```python
from build123d import *

# Parameters (mm, degrees)
CROQUIS1_W              = 30
CROQUIS1_H              = 15
CROQUIS1_W_2            = 12.5
CROQUIS1_H_2            = 12.5
SALIENTE_EXTRUIR1_DEPTH = 10
CHAFL_N1_SIZE           = 10
CHAFL_N1_SIZE2          = 2.679491924
REDONDEO1_R             = 1


with BuildPart() as part:
    # Croquis1 → Saliente-Extruir1 (new body)
    with BuildSketch(Plane(origin=(0, 0, 0), x_dir=(1, 0, 0), z_dir=(0, 1, 0))):
        with Locations((15, 7.5)):
            Rectangle(CROQUIS1_W, CROQUIS1_H)
        with Locations((7.75, 7.5)):
            Rectangle(CROQUIS1_W_2, CROQUIS1_H_2, mode=Mode.SUBTRACT)
    extrude(amount=SALIENTE_EXTRUIR1_DEPTH)

    # Chaflán1
    chafl_n1_edges = [part.edges().sort_by_distance(p)[0] for p in [
        (14, 10, -7.5),
    ]]
    chafl_n1_side = [part.faces().sort_by_distance(p)[0] for p in [
        (18.856382979, 10, -7.5),
    ]]
    chamfer(chafl_n1_edges, length=CHAFL_N1_SIZE, length2=CHAFL_N1_SIZE2, reference=chafl_n1_side[0])

    # Redondeo1
    redondeo1_edges = [part.edges().sort_by_distance(p)[0] for p in [
        (1.5, 5, -13.75),
        (1.5, 5, -1.25),
        (14, 3.660254038, -1.25),
        (14, 3.660254038, -13.75),
        (0, 5, -15),
        (0, 5, 0),
    ]]
    fillet(redondeo1_edges, radius=REDONDEO1_R)


solid = part.part
```
Input: part model. Units: mm. Frame: model coordinates. A direction names the side the tool comes from. Round coordinates to 2 decimals unless told otherwise and drop trailing zeros. Loops run counter-clockwise (first coordinate to the right, second up) from the corner with the lowest first, then second, coordinate; pieces in that order, holes last. Notation, with made-up numbers: (76, 14.5) -> (102, 14.5) arc R12 ccw to (102, 28.5) -> close; hole circle Ø2 at (41.5, -6). An arc over 180 degrees is marked (long way). Use one line per item in the form item = value. Start each with the question number.
Item 1: Section query C-C on y = 0.75. Return the cut outline in (x, z).
Item 2: Mould query, pull axis Z, two halves, no side actions, for faces 1 (the face through (15, 5, -15)), 2 (the face through (30, 5, -7)), 3 (the face through (14, 4, -7)). Classes: pulls with the +Z half, pulls with the -Z half, needs draft (parallel to the pull), parting line crosses it, or undercut.
Item 3: Section query B-B on z = -5.25. Return the cut outline in (x, y).
Item 4: Material intervals for L1, parallel to Z at x = 17, y = 9.25; L2, parallel to X at y = 7, z = -7; L3, parallel to Z at x = 13.5, y = 5, sorted ascending. Write a range as from..to.
Item 5: Section query A-A on x = 5. Return the cut outline in (y, z).
Item 6: Section query D-D on x = 17.75. Return the cut outline in (y, z).
Item 7: Set-up query: faces 4 (the face through (8, 6, -1.25)), 5 (the face through (18, 0, -8)), 6 (the face through (1.801, 5.07, -13.465)). Return all of +Z, -Z, +X, -X, +Y, -Y with unobstructed straight access to the full face (end or side cutting, diameter ignored); none if empty.
Ans:
q1.outline = (0, -14) arc R1 ccw to (1, -15) -> (30, -15) -> (30, 0) -> (1, 0) arc R1 ccw to (0, -1) -> close; hole (1.5, -12.75) arc R1 ccw to (2.5, -13.75) -> (13, -13.75) arc R1 ccw to (14, -12.75) -> (14, -2.25) arc R1 ccw to (13, -1.25) -> (2.5, -1.25) arc R1 ccw to (1.5, -2.25) -> close
q2.face_1 = pulls with the -Z half
q2.face_2 = needs draft
q2.face_3 = undercut
q3.outline = (0, 0) -> (1.5, 0) -> (1.5, 10) -> (0, 10) -> close; (14, 0) -> (30, 0) -> (30, 10) -> (24, 10) -> (14, 7.32) -> close
q4.L1 = -15..-13.75, -1.25..0
q4.L2 = 0..1.5, 14..30
q4.L3 = -15..-13.62, -1.38..0
q5.outline = (0, -15) -> (10, -15) -> (10, -13.75) -> (0, -13.75) -> close; (0, -1.25) -> (10, -1.25) -> (10, 0) -> (0, 0) -> close
q6.outline = (0, -15) -> (10, -15) -> (10, -13.75) -> (8.33, -13.75) -> (8.33, -1.25) -> (10, -1.25) -> (10, 0) -> (0, 0) -> close
q7.face_4 = +Y
q7.face_5 = +Z, -Z, +X, -X, -Y
q7.face_6 = +Y, -Y
